Source: CAD feature listing. Evaluate the final solid. Frame: model axes, mm. A direction names the side the tool comes from. Give positions to 0.01 mm unless a question says otherwise; leave off trailing zeros. Order: outer loops, then holes, each group sorted by start corner. A loop starts at its lowest first (then second) coordinate and runs counter-clockwise, first axis right, second up. Notation, with made-up numbers: (-3, -38) -> (54, -38) arc R15 cw to (54, -26) -> close; hole circle Ø7 at (-40, 22.25). An arc over 180 degrees is marked (long way). Answer in a Markdown table with one row per item.
```python
from build123d import *

# Parameters (mm, degrees)
F0_W     = 283.9974
F0_H     = 76.2
F1_DEPTH = 38.1
F4_R     = 2.794
F3_R     = 2.794
F5_DEPTH = 38.101
F2_W     = 82.55
F2_H     = 76.2
F6_DEPTH = 22.86


with BuildPart() as f1:
    # F0 (on Top) → F1 (new body)
    with BuildSketch(Plane.XY):
        with Locations((141.9987, -38.1)):
            Rectangle(F0_W, F0_H)
    extrude(amount=-F1_DEPTH)

    # F4 (on face) + F3 (on face) → F5 (cut, through all)
    with BuildSketch(Plane(origin=(0, 0, -38.1), x_dir=(1, 0, 0), z_dir=(0, 0, -1))):
        with Locations((279.2222, 15.875)):
            Circle(F4_R)
        with Locations((279.2222, 60.325)):
            Circle(F4_R)
        with Locations((206.1972, 60.325)):
            Circle(F4_R)
        with Locations((206.1972, 15.875)):
            Circle(F4_R)
    with BuildSketch(Plane(origin=(0, 0, -38.1), x_dir=(1, 0, 0), z_dir=(0, 0, -1))):
        with Locations((77.8002, 60.325)):
            Circle(F3_R)
        with Locations((77.8002, 15.875)):
            Circle(F3_R)
        with Locations((4.7752, 15.875)):
            Circle(F3_R)
        with Locations((4.7752, 60.325)):
            Circle(F3_R)
    extrude(amount=-F5_DEPTH, mode=Mode.SUBTRACT)

    # F2 (on face) → F6 (cut)
    with BuildSketch(Plane(origin=(0, 0, -38.1), x_dir=(1, 0, 0), z_dir=(0, 0, -1))):
        with Locations((41.275, 38.1)):
            Rectangle(F2_W, F2_H)
        with Locations((242.7224, 38.1)):
            Rectangle(F2_W, F2_H)
    extrude(amount=-F6_DEPTH, mode=Mode.SUBTRACT)


solid = f1.part
```
(1) Ray query, probe 1 along Y at (x, z) = (207.5, -7.5); probe 2 along X at (y, z) = (-59.5, -33); probe 3 along Z at (x, y) = (259, -16.5). Return the intervals inside material, ascending.
A:
| item | result |
|---|---|
| probe 1 | y = -76.2 to -62.8, -57.85 to -18.35, -13.4 to 0 |
| probe 2 | x = 82.55 to 201.45 |
| probe 3 | z = -15.24 to 0 |
(2) Section query B-B (z = -34.5). Return the cut outline in (x, y), plus the area to 3 significant figures.
A:
| item | result |
|---|---|
| outline | (82.55, -76.2) -> (201.45, -76.2) -> (201.45, 0) -> (82.55, 0) -> close |
| area | 9,060 mm^2 |
(3) Pull-direction query (X, two-part tool) for faces 4 (the flat face through (140, -76.2, -15)), 5 (the flat face through (82.55, -38, -27)), 6 (the cylindrical face through (204, -58.6, -7.7)); classes: +X half, -X half, draft (parallel to the pull), parting line (faces both ways), or undercut.
A:
| item | result |
|---|---|
| face 4 | draft |
| face 5 | -X half |
| face 6 | undercut |
(4) First-contact query: pin 1 Ø23 at (x, y) = (54, -47) entering from -Z; pin 2 Ø11.5 at (y, z) = (-24, -24.5) entering from +X; pin 3 Ø3.5 at (x, y) = (4.78, -15.88) entering from +Z. Flat tips, straight axial feed; report the tip coordinate or a pass-through.
A:
| item | result |
|---|---|
| pin 1 | stops at z = -15.24 |
| pin 2 | stops at x = 201.45 |
| pin 3 | passes through |
(5) Access query for faces 1 (the flat face through (41, -39, -15.24)), 2 (the flat face through (283.997, -39, -8)), 3 (the flat face through (201.447, -38, -27)). Directions: +Z, -Z, +X, -X, +Y, -Y. A direction counts if a zero-diameter tool reaches every point of the face in a straight line with its end or side. Return the directions, or none.
A:
| item | result |
|---|---|
| face 1 | -Z, -X, +Y, -Y |
| face 2 | +Z, -Z, +X, +Y, -Y |
| face 3 | -Z, +X, +Y, -Y |
(6) Section query A-A (y = -69). Return the cut outline in (x, z), plus the area to 3 significant figures.
A:
| item | result |
|---|---|
| outline | (0, -15.24) -> (82.55, -15.24) -> (82.55, -38.1) -> (201.45, -38.1) -> (201.45, -15.24) -> (284, -15.24) -> (284, 0) -> (0, 0) -> close |
| area | 7,050 mm^2 |
(7) Section query C-C (x = 56). Return the cut outline in (y, z).
A:
| item | result |
|---|---|
| outline | (-76.2, -15.24) -> (0, -15.24) -> (0, 0) -> (-76.2, 0) -> close |
